Verification items for the finished model (mm, model axes). Face numbers are marked on the shaded views. A direction names the side the tool comes from. Round coordinates to 2 decimals unless told otherwise and drop trailing zeros. Order: outer loops, then holes, each group sorted by start corner. A loop starts at its lowest first (then second) coordinate and runs counter-clockwise, first axis right, second up. Notation, with made-up numbers: M -30.5,-21 L 10.5,-21 A14 ccw 10.5,-5 Z; hole C -6,35 d9. An arc over 180 degrees is marked long. One line per item, written item: value. Start each with the question number.
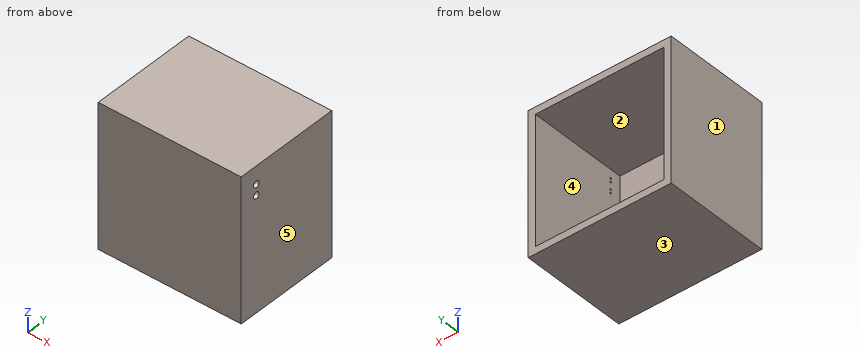
from build123d import *

# Parameters (mm, degrees)
SKETCH1_W           = 101.6
SKETCH1_H           = 101.6
BOSS_EXTRUDE1_DEPTH = 76.2
SKETCH2_W           = 91.44
SKETCH2_H           = 91.44
CUT_EXTRUDE1_DEPTH  = 71.12
SKETCH3_R           = 2.38125
CUT_EXTRUDE2_DEPTH  = 2.54
SKETCH4_R           = 0.635
CUT_EXTRUDE3_DEPTH  = 2.54
SKETCH6_R           = 2.38125
CUT_EXTRUDE5_DEPTH  = 2.54
SKETCH8_R           = 0.635
CUT_EXTRUDE7_DEPTH  = 2.54


with BuildPart() as part:
    # Sketch1 → Boss-Extrude1 (new body)
    with BuildSketch(Plane(origin=(0, 0, 0), x_dir=(1, 0, 0), z_dir=(0, 1, 0))):
        with Locations((-46.892307692, 7.947401247)):
            Rectangle(SKETCH1_W, SKETCH1_H)
    extrude(amount=BOSS_EXTRUDE1_DEPTH)

    # Sketch2 → Cut-Extrude1 (cut)
    with BuildSketch(Plane(origin=(0, 76.2, 0), x_dir=(1, 0, 0), z_dir=(0, 1, 0))):
        with Locations((-46.892307692, 7.947401247)):
            Rectangle(SKETCH2_W, SKETCH2_H)
    extrude(amount=-CUT_EXTRUDE1_DEPTH, mode=Mode.SUBTRACT)

    # Sketch3 → Cut-Extrude2 (cut)
    with BuildSketch(Plane(origin=(3.907692308, 0, 0), x_dir=(0, 0, -1), z_dir=(1, 0, 0))):
        with Locations((-30.152598753, 12.7)):
            Circle(SKETCH3_R)
    extrude(amount=-CUT_EXTRUDE2_DEPTH, mode=Mode.SUBTRACT)

    # Sketch4 → Cut-Extrude3 (cut)
    with BuildSketch(Plane(origin=(1.367692308, 0, 0), x_dir=(0, 0, -1), z_dir=(1, 0, 0))):
        with Locations((-31.42844237, 12.756924018)):
            Circle(SKETCH4_R)
        with Locations((-28.88844237, 12.859462566)):
            Circle(SKETCH4_R)
    extrude(amount=-CUT_EXTRUDE3_DEPTH, mode=Mode.SUBTRACT)

    # Sketch6 → Cut-Extrude5 (cut)
    with BuildSketch(Plane(origin=(3.907692308, 0, 0), x_dir=(0, 0, -1), z_dir=(1, 0, 0))):
        with Locations((-22.532598753, 12.7)):
            Circle(SKETCH6_R)
    extrude(amount=-CUT_EXTRUDE5_DEPTH, mode=Mode.SUBTRACT)

    # Sketch8 → Cut-Extrude7 (cut)
    with BuildSketch(Plane(origin=(1.367692308, 0, 0), x_dir=(0, 0, -1), z_dir=(1, 0, 0))):
        with Locations((-23.822454546, 12.843688335)):
            Circle(SKETCH8_R)
        with Locations((-21.299543609, 12.843688335)):
            Circle(SKETCH8_R)
    extrude(amount=-CUT_EXTRUDE7_DEPTH, mode=Mode.SUBTRACT)


solid = part.part
1. Section check B-B (z = 11). Record the cut outline in (x, y), and give its area (3 significant figures).
2. Draft check along Z on the marked faces 3, 4 and 5. Enter one of: released by +Z, released by -Z, zero draft, split by the parting line, or undercut.
3. Scan lines: line 1 along X through (y, z) = (44, -25.5); line 2 along Z through (x, y) = (-79, 26.5); line 3 along Y through (x, z) = (-62, -50). Record each from-to range of solid material in increasing order.
4. Section check C-C (x = -64.5). Record the cut outline in (y, z), and give its area (3 significant figures).
5. Depth check by flat-ended pin: pin 1 (4 mm diameter, centred on y = 12.7, z = 22.53, fed in from +X); pin 2 (0.8 mm diameter, centred on y = 12.86, z = 28.89, fed in from +X). Enter the tip coordinate at first touch or a pass-through.
6. Tool access check on the marked faces 1 and 2. Record the directions out of +Z, -Z, +X, -X, +Y, -Y that give a thin tool (end or side, any length) a straight path to the whole face; none if there is none.
7. Section check A-A (y = 40). Record the cut outline in (x, z), and give its area (3 significant figures).
Geometry check:
1. outline: M -97.69,0 L 3.91,0 L 3.91,76.2 L -1.17,76.2 L -1.17,5.08 L -92.61,5.08 L -92.61,76.2 L -97.69,76.2 Z
1. area: 1,240 mm²
2. face 3: released by -Z
2. face 4: undercut
2. face 5: zero draft
3. line 1: x = -97.69 to -92.61, -1.17 to 3.91
3. line 2: z = -58.75 to -53.67, 37.77 to 42.85
3. line 3: y = 0 to 5.08
4. outline: M 0,-58.75 L 76.2,-58.75 L 76.2,-53.67 L 5.08,-53.67 L 5.08,37.77 L 76.2,37.77 L 76.2,42.85 L 0,42.85 Z
4. area: 1,240 mm²
5. pin 1: stops at x = 1.37
5. pin 2: stops at x = -92.61
6. face 1: +Z, -Z, -X, +Y, -Y
6. face 2: +Y
7. outline: M -97.69,-58.75 L 3.91,-58.75 L 3.91,42.85 L -97.69,42.85 Z; hole M -92.61,-53.67 L -1.17,-53.67 L -1.17,37.77 L -92.61,37.77 Z
7. area: 1,960 mm²
